```python
from build123d import *

# Parameters (mm, degrees)
F1_DEPTH = 330.2
F2_W     = 294.132
F2_H     = 357.632
F3_DEPTH = 25.4
F4_R     = 130.175
F5_DEPTH = 10.16
F6_W     = 294.132
F6_H     = 25.4
F7_DEPTH = 25.4


with BuildPart() as f1:
    # F0 (on Right) → F1 (new body)
    with BuildSketch(Plane.YZ):
        Polygon((85.2122760074, 384.3677380031), (0, 0), (364.2337952902, 0), (432.3831361393, 307.4018112867), align=None)
    extrude(amount=F1_DEPTH)

    # F2 (on face) → F3 (cut)
    with BuildSketch(Plane(origin=(0, 0, 0), x_dir=(1, 0, 0), z_dir=(0, -0.9762960071, 0.2164396139))):
        with Locations((165.1, 196.85)):
            Rectangle(F2_W, F2_H)
    extrude(amount=-F3_DEPTH, mode=Mode.SUBTRACT)

    # F4 (on face) → F5 (join)
    with BuildSketch(Plane(origin=(0, 24.7979185808, -5.497566194), x_dir=(1, 0, 0), z_dir=(0, -0.9762960071, 0.2164396139))):
        with Locations((165.1, 210.566)):
            Circle(F4_R)
    extrude(amount=F5_DEPTH)

    # F6 (on face) → F7 (cut)
    with BuildSketch(Plane(origin=(0, 24.7979185808, -5.497566194), x_dir=(1, 0, 0), z_dir=(0, -0.9762960071, 0.2164396139))):
        with Locations((165.1, 30.734)):
            Rectangle(F6_W, F6_H)
    extrude(amount=-F7_DEPTH, mode=Mode.SUBTRACT)


solid = f1.part
```
CAD build for the part. Positions are in the model's coordinates, mm. A direction names the side the tool comes from. Round coordinates to 2 decimals unless told otherwise and drop trailing zeros. Order: outer loops, then holes, each group sorted by start corner. A loop starts at its lowest first (then second) coordinate and runs counter-clockwise, first axis right, second up.
Item 1: Pin check, flat tips, straight feed: pin 1 (4 mm diameter, centred on x = 239, z = 338.5, fed in from -Y); pin 2 (2 mm diameter, centred on x = 108.5, z = 197.5, fed in from -Y); pin 3 (2 mm diameter, centred on x = 230.5, y = 230.5, fed in from +Z). Stop position of each tip, or through.
Item 2: Saw through at C-C on y = 151. Write the cut outline in (x, z), then the cut area to 3 significant figures.
Item 3: Saw through at A-A on x = 260. Write the cut outline in (y, z), then the cut area to 3 significant figures.
Item 4: Mould opens along X. For faces 4 (the face through (0, 213, 195)), 5 (the face through (312.166, 55, 187)), 6 (the face through (162.79, 397.83, 151.55)) say: pulls with the +X half, pulls with the -X half, needs draft (parallel to the pull), parting line crosses it, or undercut.
Item 5: Tool access for faces 1 (the face through (163.041, 56.286, 19.184)), 2 (the face through (17.574, 42.805, 193.081)), 3 (the face through (163.04, 93.53, 364.05)): list every direction of +Z, -Z, +X, -X, +Y, -Y with a clear straight run to the whole face (end or side of a thin tool).
Item 6: Saw through at D-D on y = 299.5. Write the cut outline in (x, z).
Item 7: Probe line 1 along Z through (x, y) = (69, 329); line 2 along Y through (x, z) = (315, 24); line 3 along Y through (x, z) = (44, 181). List the from-to ranges inside material, lowest first.
Item 8: Saw through at B-B on x = 156.5. Write the cut outline in (y, z), then the cut area to 3 significant figures.
Reported:
1. pin 1: stops at y = 100.62
1. pin 2: stops at y = 59.17
1. pin 3: stops at z = 352.38
2. outline: (0, 0) - (330.2, 0) - (330.2, 369.78) - (0, 369.78) - close
2. area: 122,000 mm2
3. outline: (0, 0) - (364.23, 0) - (432.38, 307.4) - (85.21, 384.37) - (81.31, 366.76) - (106.11, 361.26) - (89.66, 287.07) - (79.74, 289.27) - (41.17, 115.28) - (51.09, 113.09) - (34.2, 36.91) - (59, 31.41) - (53.5, 6.61) - (3.9, 17.61) - close
3. area: 118,000 mm2
4. face 4: pulls with the -X half
4. face 5: undercut
4. face 6: needs draft
5. face 1: none
5. face 2: +Z, +X, -X, -Y
5. face 3: -Y
6. outline: (0, 0) - (330.2, 0) - (330.2, 336.86) - (0, 336.86) - close
7. line 1: z = 0 to 330.32
7. line 2: y = 5.32 to 369.55
7. line 3: y = 55.74 to 404.36
8. outline: (0, 0) - (364.23, 0) - (432.38, 307.4) - (85.21, 384.37) - (81.31, 366.76) - (106.11, 361.26) - (98.49, 326.89) - (88.57, 329.09) - (32.34, 75.46) - (42.26, 73.27) - (34.2, 36.91) - (59, 31.41) - (53.5, 6.61) - (3.9, 17.61) - close
8. area: 119,000 mm2
